Here's how the part is built. I have some questions about the finished solid (model axes, mm). A direction names the side the tool comes from. Round coordinates to 2 decimals unless told otherwise and drop trailing zeros. Loops run counter-clockwise (first coordinate to the right, second up) from the corner with the lowest first, then second, coordinate; pieces in that order, holes last. Notation, with made-up numbers: (8.5, -33.5) -> (60.5, -33.5) arc R35 ccw to (60.5, -1.5) -> close; hole circle Ø6 at (61.25, 7). An arc over 180 degrees is marked (long way). Use one line per item in the form item = value. Start each with the question number.
Item 1: If we section it at C-C (x = -18.5): Write out the boundary of the cut face in (y, z) (1 decimal), then the cut area to 3 significant figures.
Item 2: If I drill on L1, parallel to Y at x = 33.2, z = 0; L2, parallel to X at y = 11, z = 0; L3, parallel to Y at x = -32.9, z = 0, over which ranges is the centre line in solid material (lowest first)? Write a range as [from, to].
Item 3: I'm going to push flat-ended pins straight in: pin 1 Ø3 at (y, z) = (-3.5, 2.5) entering from -X; pin 2 Ø6 at (x, z) = (-11, 3) entering from -Y; pin 3 Ø3.5 at (x, z) = (10, -2.5) entering from +Y. Where does each tip first touch, or does it pass through?
Item 4: If we section it at B-B (y = 7.25): Write out the boundary of the cut face in (x, z), then the cut area to 3 significant figures.
Item 5: For faces 1 (the face through (5, 8, -4.76)), 2 (the face through (10.453, -0.022, -3.198)), 3 (the face through (-36, -5, 0)), 4 (the face through (36, -5, 0)), 5 (the face through (-33.465, -5.175, 0.186)), which set-ups out of +Z, -Z, +X, -X, +Y, -Y let a thin tool reach every point of the face, with its end or its side?
Item 6: If we section it at A-A (y = -3.25): Write out the boundary of the cut face in (x, z) (3 decimals).
Item 7: Thinking about a two-plate mould opening in X: for faces 6 (the face through (-4.76, 0, 0)), 7 (the face through (-4.755, 11.181, 0.209)), 8 (the face through (0, 0, 5.675)), which applies, released by +X, released by -X, zero draft, split by the parting line, or undercut?
Solid Edge part; units mm, degrees
sketch "Sketch1" plane through (0, 0, 0) normal (0, -1, 0) x (1, 0, 0)
  line L0 (-41, -7.5) -> (41, -7.5)
  line L1 (41, -7.5) -> (41, 7.5)
  line L2 (41, 7.5) -> (-41, 7.5)
  line L3 (-41, 7.5) -> (-41, -7.5)
  dimension "D1" = 41
  dimension "D2" = 41
extrude "Protrusion1" add sketch "Sketch1" along normal mid plane 3.175
sketch "Sketch2" plane through (0, -1.5875, 0) normal (0, -1, 0) x (1, 0, 0)
  line L0 (-36, -3.175) -> (-31, -3.175)
  line L1 (-31, -3.175) -> (-31, 3.175)
  line L2 (-31, 3.175) -> (-36, 3.175)
  line L3 (-36, 3.175) -> (-36, -3.175)
  line L4 (36, -3.175) -> (31, -3.175)
  line L5 (31, -3.175) -> (31, 3.175)
  line L6 (31, 3.175) -> (36, 3.175)
  line L7 (36, 3.175) -> (36, -3.175)
  dimension "D1" = 31
  dimension "D2" = 36
extrude "ExtrudedProtrusion_2" add sketch "Sketch2" along normal blind 8.17
extrude "Cutout1" [suppressed]
hole "Hole_1" at (0, -6.5875, 0) direction (-1, 0, 0) diameter 2.85 end through all thread major 3.5 thread length 2
hole "Hole_2" at (0, -6.5875, 0) direction (1, 0, 0) diameter 2.459 end through all thread major 3 thread length 2
sketch "Sketch3" plane through (0, 1.5875, 0) normal (0, 1, 0) x (1, 0, 0)
  circle A0 centre (0, 0) radius 4.76
extrude "ExtrudedProtrusion_3" add sketch "Sketch3" along normal blind 15.88
sketch "Sketch4" plane through (0, 1.5875, 0) normal (0, 1, 0) x (1, 0, 0)
  line L0 (10, 4.76) -> (0, 4.76)
  line L1 (0, 4.76) -> (0, -4.76)
  line L2 (0, -4.76) -> (10, -4.76)
  line L3 (10, -4.76) -> (10, 4.76)
  dimension "D1" = 10
  dimension "D2" = 10
extrude "ExtrudedProtrusion_4" add sketch "Sketch4" along normal blind 12.88
fillet "Round_1" radius 1 2 edges at (10, 8.0275, -4.76) (10, 8.0275, 4.76)
hole "Hole_3" at (0, 17.4675, 0) direction (0, -1, 0) diameter 3.9675 end through all thread major 4.826 thread length 2
chamfer "Chamfer_1" distance 3 angle 45 4 edges at (41, 0, 7.5) (41, 0, -7.5) (-41, 0, 7.5) (-41, 0, -7.5)
fillet "Round_2" radius 3.175 4 edges at (-33.5, -9.7575, -3.175) (-33.5, -9.7575, 3.175) (33.5, -9.7575, 3.175) (33.5, -9.7575, -3.175)
sketch "Sketch5" plane through (0, -1.5875, 0) normal (0, -1, 0) x (1, 0, 0)
  line L0 (-38.5, -5.675) -> (38.5, -5.675)
  line L1 (38.5, -5.675) -> (38.5, 5.675)
  line L2 (38.5, 5.675) -> (-38.5, 5.675)
  line L3 (-38.5, 5.675) -> (-38.5, -5.675)
  line L4 (43.8094, 8.6849) -> (-43.8094, 8.6849)
  line L5 (-43.8094, 8.6849) -> (-43.8094, -8.6849)
  line L6 (-43.8094, -8.6849) -> (43.8094, -8.6849)
  line L7 (43.8094, -8.6849) -> (43.8094, 8.6849)
extrude "Cutout2" cut sketch "Sketch5" against normal up to surface (3.175 mm away)
sketch "Sketch6" plane through (0, 1.5875, 0) normal (0, 1, 0) x (-1, 0, 0)
  line L0 (31, 3.675) -> (4.76, 3.675)
  line L1 (4.76, 3.675) -> (4.76, -3.675)
  line L2 (4.76, -3.675) -> (31, -3.675)
  line L3 (31, -3.675) -> (31, 3.675)
  line L4 (-31, 3.675) -> (-10, 3.675)
  line L5 (-10, 3.675) -> (-10, -3.675)
  line L6 (-10, -3.675) -> (-31, -3.675)
  line L7 (-31, -3.675) -> (-31, 3.675)
  dimension "D1" = 31
extrude "Cutout3" cut sketch "Sketch6" against normal up to surface (3.175 mm away)
fillet "Round_5" radius 1.5875 4 edges at (10, 0, -3.675) (10, 0, 3.675) (-4.76, 0, -3.675) (-4.76, 0, 3.675)
chamfer "Chamfer_2" distance 3 angle 45 4 edges at (38.5, 0, -5.675) (38.5, 0, 5.675) (-38.5, 0, 5.675) (-38.5, 0, -5.675)
properties material "Aluminium, 6061-T6"
Values found:
q1.outline = (-1.6, -5.7) -> (1.6, -5.7) -> (1.6, -3.7) -> (-1.6, -3.7) -> close; (-1.6, 3.7) -> (1.6, 3.7) -> (1.6, 5.7) -> (-1.6, 5.7) -> close
q1.area = 12.7 mm2
q2.L1 = [-9.76, -7.82], [-5.36, 1.59]
q2.L2 = [-4.76, -1.98], [1.98, 10]
q2.L3 = [-9.76, -8.01], [-5.16, 1.59]
q3.pin_1 = -36
q3.pin_2 = -1.59
q3.pin_3 = 14.47
q4.outline = (0, -4.76) -> (9, -4.76) arc R1 ccw to (10, -3.76) -> (10, 3.76) arc R1 ccw to (9, 4.76) -> (0, 4.76) arc R4.76 ccw to start; hole circle Ø3.97 at (0, 0)
q4.area = 118 mm2
q5.face_1 = -Z, +X, -X, +Y
q5.face_2 = +Y, -Y
q5.face_3 = +Z, -Z, -X, -Y
q5.face_4 = +Z, -Z, +X, -Y
q5.face_5 = -X
q6.outline = (-36, -3.175) -> (-31, -3.175) -> (-31, 3.175) -> (-36, 3.175) -> close; (31, -3.175) -> (36, -3.175) -> (36, 3.175) -> (31, 3.175) -> close
q7.face_6 = undercut
q7.face_7 = split by the parting line
q7.face_8 = zero draft
